The listing builds one solid part. Answer for the finished solid, in the listing's coordinates (mm). A direction names the side the tool comes from. Round coordinates to 2 decimals unless told otherwise and drop trailing zeros. Write each loop counter-clockwise with the first axis right and the second up, starting at its lowest first coordinate (ties: lowest second). Pieces come first, ordered by that corner, then holes.
(1) The mould has two halves that part along Y. Classify faces 5 (the face through (-42.637, -0.754, 0.74)), 6 (the face through (-25.637, -0.754, 0.74)), 7 (the face through (-33, 0, 0)), 8 (the face through (-21.041, -3.907, 0.74)): +Y half, -Y half, draft (parallel to the pull), parting line (faces both ways), or undercut.
(2) A cutting plane is placed at C-C, the plane y = -4.5. Give the vertices of the cut face in (x, z), and give its area (3 significant figures).
(3) For faces 1 (the face through (-25, 3.452, 1)), 2 (the face through (-40.638, -8, 1)), 3 (the face through (-40.638, 8, 1)), 4 (the face through (-25, -5.048, 1)), determine the directions among +Z, -Z, +X, -X, +Y, -Y from which every point of the face is accessible in a straight line to the end or side of a thin tool.
(4) A cutting plane is placed at B-B, the plane y = -7. Give the vertices of the cut face in (x, z).
(5) A cutting plane is placed at A-A, the plane z = 0.7. Give the vertices of the cut face in (x, y), and give its area (3 significant figures).
(6) Find the intervals of material crossed by probe 1 along X at (y, z) = (-0.75, 0.1); probe 2 along X at (y, z) = (5.5, 0.9); probe 3 along Y at (x, z) = (-41, 0.45), in increasing order.
from build123d import *

# Parameters (mm, degrees)
ESBO_O2_W                = 28.244172386
ESBO_O2_H                = 13.944205314
RESSALTO_EXTRUS_O1_DEPTH = 2.54
ESBO_O3_R                = 1
RESSALTO_EXTRUS_O2_DEPTH = 1.5
ESBO_O4_W                = 28.244172386
ESBO_O4_H                = 13.944205314
CORTE_EXTRUS_O1_DEPTH    = 2.54


with BuildPart() as part:
    # Esboço2 → Ressalto-extrusão1 (new body)
    with BuildSketch(Plane.XY):
        Rectangle(ESBO_O2_W, ESBO_O2_H)
    extrude(amount=RESSALTO_EXTRUS_O1_DEPTH)

    # Esboço4 → Corte-extrusão1 (cut)
    with BuildSketch(Plane.XY.offset(2.54)):
        Rectangle(ESBO_O4_W, ESBO_O4_H)
    extrude(amount=-CORTE_EXTRUS_O1_DEPTH, mode=Mode.SUBTRACT)


with BuildPart() as body_2:
    # Esboço3 → Ressalto-extrusão2 (new body)
    with BuildSketch(Plane.XY):
        with BuildLine():
            Line((-40.638175932, 11.952156585), (-40.638175932, 3.452156585))
            Line((-40.638175932, 3.452156585), (-42.438175932, 3.452156585))
            ThreePointArc((-42.438175932, 3.452156585), (-45.266603057, 2.28058371), (-46.438175932, -0.547843415))
            Line((-46.438175932, -0.547843415), (-46.438175932, -1.047843415))
            ThreePointArc((-46.438175932, -1.047843415), (-45.266603057, -3.876270539), (-42.438175932, -5.047843415))
            Line((-42.438175932, -5.047843415), (-40.638175932, -5.047843415))
            Line((-40.638175932, -5.047843415), (-40.638175932, -12.047843415))
            Line((-40.638175932, -12.047843415), (-25.638175932, -12.047843415))
            Line((-25.638175932, -12.047843415), (-25.638175932, -5.047843415))
            Line((-25.638175932, -5.047843415), (-23.838175932, -5.047843415))
            ThreePointArc((-23.838175932, -5.047843415), (-21.009748807, -3.876270539), (-19.838175932, -1.047843415))
            Line((-19.838175932, -1.047843415), (-19.838175932, -0.547843415))
            ThreePointArc((-19.838175932, -0.547843415), (-21.009748807, 2.28058371), (-23.838175932, 3.452156585))
            Line((-23.838175932, 3.452156585), (-25.638175932, 3.452156585))
            Line((-25.638175932, 3.452156585), (-25.638175932, 11.952156585))
            Line((-25.638175932, 11.952156585), (-40.638175932, 11.952156585))
        make_face()
        with Locations((-41.638175932, -0.797843415)):
            Circle(ESBO_O3_R, mode=Mode.SUBTRACT)
        with Locations((-24.638175932, -0.797843415)):
            Circle(ESBO_O3_R, mode=Mode.SUBTRACT)
    extrude(amount=RESSALTO_EXTRUS_O2_DEPTH)


solid = body_2.part
Solutions:
1. face 5: undercut
1. face 6: undercut
1. face 7: draft
1. face 8: -Y half
2. outline: (-44.46, 0) - (-21.82, 0) - (-21.82, 1.5) - (-44.46, 1.5) - close
2. area: 34.0 mm2
3. face 1: +Z, -Z, +X, +Y
3. face 2: +Z, -Z, -X, -Y
3. face 3: +Z, -Z, -X, +Y
3. face 4: +Z, -Z, +X, -Y
4. outline: (-40.64, 0) - (-25.64, 0) - (-25.64, 1.5) - (-40.64, 1.5) - close
5. outline: (-46.44, -1.05) arc R4 ccw to (-42.44, -5.05) - (-40.64, -5.05) - (-40.64, -12.05) - (-25.64, -12.05) - (-25.64, -5.05) - (-23.84, -5.05) arc R4 ccw to (-19.84, -1.05) - (-19.84, -0.55) arc R4 ccw to (-23.84, 3.45) - (-25.64, 3.45) - (-25.64, 11.95) - (-40.64, 11.95) - (-40.64, 3.45) - (-42.44, 3.45) arc R4 ccw to (-46.44, -0.55) - close; hole circle Ø2 at (-41.64, -0.8); hole circle Ø2 at (-24.64, -0.8)
5. area: 439 mm2
6. probe 1: x = -46.44 to -42.64, -40.64 to -25.64, -23.64 to -19.84
6. probe 2: x = -40.64 to -25.64
6. probe 3: y = -5.05 to -1.57, -0.03 to 3.45
